CAD build for the part. Positions are in the model's coordinates, mm. A direction names the side the tool comes from. Coordinates: 2 decimals unless noted, no trailing zeros. Write each loop counter-clockwise with the first axis right and the second up, starting at its lowest first coordinate (ties: lowest second). Pieces come first, ordered by that corner, then holes. Notation, with made-up numbers: (81.25, 84.25) - (106.25, 84.25) arc R18 ccw to (106.25, 99.25) - close; hole circle Ø9 at (25, 47.25). An arc over 180 degrees is marked (long way). Answer in a Markdown table with one row per item. Add a question column.
Q1. 3-axis set-ups, long thin cutter, end or side, ignore diameter. For faces 1 (the flat face through (199, 0, 917)), 2 (the flat face through (373, 123, 1040)): which of +Z, -Z, +X, -X, +Y, -Y reach the whole face in a straight line?
Q2. Two-plate mould, pull along Z, no slides. Class faces 3 (the flat face through (203, 296, 1700)), 4 (the flat face through (101, 296, 200)), 5 (the flat face through (199, 600, 854)): +Z half, -Z half, draft (parallel to the pull), parting line (faces both ways), or undercut.
Q3. Band-saw the part on C-C (y = 512). State how many separate pieces and enclosed holes the cut face has, and give its area (3 significant figures).
Q4. Band-saw the part on A-A (x = 293). List the corners of the cut face in (y, z), and give its area (3 significant figures).
Q5. Band-saw the part on B-B (z = 1497.5). List the corners of the cut face in (x, y).
Q6. Pin check, flat tips, straight feed: pin 1 (1 mm diameter, centred on y = 376.5, z = 1068.5, fed in from -X); pin 2 (5 mm diameter, centred on x = 377, z = 545, fed in from +Y). Stop position of each tip, or through.
Q7. Drill centre lines: line 1 along Z through (x, y) = (384, 430.5); line 2 along X through (y, z) = (566, 227.5); line 3 along Z through (x, y) = (309.5, 558.5). Where is each one in solid material? Low to high. Write a range as from..to.
Autodesk Inventor part; units mm, degrees
ref_plane "YZ Plane" through (0, 0, 0) normal (1, 0, 0) x (0, 1, 0)
ref_plane "XZ Plane" through (0, 0, 0) normal (0, 1, 0) x (-1, 0, 0)
ref_plane "XY Plane" through (0, 0, 0) normal (0, 0, 1) x (1, 0, 0)
sketch "Sketch2" plane through (0, 0, 0) normal (0, 1, 0) x (-1, 0, 0)
  line L0 (-400, 180) -> (-400, 1700)
  line L1 (-400, 1700) -> (0, 1700)
  line L2 (0, 1700) -> (0, 180)
  line L3 (-400, 200) -> (-400, 600)
  line L4 (0, 600) -> (0, 200)
  line L5 (0, 600) -> (0, 700)
  line L6 (-400, 700) -> (-400, 600)
  line L7 (-400, 700) -> (-400, 1100)
  line L8 (0, 1100) -> (0, 700)
  line L9 (0, 1100) -> (0, 1200)
  line L10 (-400, 1200) -> (-400, 1100)
  line L11 (-400, 1200) -> (-400, 1600)
  line L12 (0, 1600) -> (0, 1200)
  line L13 (0, 200) -> (0, 180)
  line L14 (0, 180) -> (-400, 180)
  line L15 (-400, 180) -> (-400, 200)
  line L16 (0, 700) -> (0, 680)
  line L17 (-400, 680) -> (-400, 700)
  line L18 (0, 1200) -> (0, 1180)
  line L19 (-400, 1180) -> (-400, 1200)
  line L20 (-390, 200) -> (-210, 200)
  line L21 (-190, 200) -> (-10, 200)
  line L22 (-10, 200) -> (-190, 200)
  line L23 (-210, 200) -> (-390, 200)
  line L24 (-210, 680) -> (-210, 200)
  line L25 (-190, 680) -> (-190, 200)
  line L26 (-390, 700) -> (-210, 700)
  line L27 (-190, 700) -> (-10, 700)
  line L28 (-10, 700) -> (-190, 700)
  line L29 (-210, 700) -> (-390, 700)
  line L30 (-10, 700) -> (-190, 700)
  line L31 (-210, 700) -> (-390, 700)
  line L32 (-10, 680) -> (-190, 680)
  line L33 (-210, 680) -> (-390, 680)
  line L34 (-10, 680) -> (-10, 200)
  line L35 (-390, 200) -> (-390, 680)
  line L36 (-210, 1690) -> (-210, 1200)
  line L37 (-210, 1180) -> (-210, 700)
  line L38 (-190, 1690) -> (-190, 1200)
  line L39 (-190, 1180) -> (-190, 700)
  line L40 (-390, 1200) -> (-210, 1200)
  line L41 (-190, 1200) -> (-10, 1200)
  line L42 (-10, 1200) -> (-190, 1200)
  line L43 (-210, 1200) -> (-390, 1200)
  line L44 (-10, 1200) -> (-190, 1200)
  line L45 (-210, 1200) -> (-390, 1200)
  line L46 (-10, 1180) -> (-190, 1180)
  line L47 (-210, 1180) -> (-390, 1180)
  line L48 (-10, 1690) -> (-10, 1200)
  line L49 (-10, 1180) -> (-10, 700)
  line L50 (-390, 700) -> (-390, 1180)
  line L51 (-390, 1200) -> (-390, 1690)
  line L52 (-390, 1690) -> (-210, 1690)
  line L53 (-190, 1690) -> (-10, 1690)
  point P0 (0, 0)
  dimension "d0" = 400
  dimension "d6" = 400
  dimension "d7" = 100
  dimension "d8" = 400
  dimension "d9" = 400
  dimension "d10" = 100
  dimension "d11" = 400
  dimension "d12" = 400
  dimension "d14" = 400
  dimension "d15" = 20
  dimension "d16" = 20
  dimension "d17" = 20
  dimension "d25" = 10
extrude "Extrusion1" add sketch "Sketch2" along normal blind 600
sketch "Sketch3" plane through (400, 0, 180) normal (0, 0, -1) x (-1, 0, 0)
  line L0 (0, 0) -> (400, 0)
  line L1 (400, 0) -> (400, 600)
  line L2 (400, 600) -> (0, 600)
  line L3 (0, 600) -> (0, 0)
  line L4 (20, 300) -> (380, 300)
  line L5 (200, 0) -> (200, 600)
  line L6 (0, 0) -> (20, 0)
  line L7 (20, 0) -> (20, 600)
  line L8 (20, 600) -> (0, 600)
  line L9 (0, 600) -> (0, 0)
  line L10 (400, 600) -> (380, 600)
  line L11 (380, 600) -> (380, 0)
  line L12 (380, 0) -> (400, 0)
  line L13 (400, 0) -> (400, 600)
  dimension "d20" = 20
  dimension "d21" = 20
extrude "Extrusion2" add sketch "Sketch3" along normal blind 200 contours L3 L2 L7 L0 | L11 L2 L1 L0
sketch "Sketch4" plane through (10, 0, 680) normal (1, 0, 0) x (0, 0, -1)
  line L0 (0, 0) -> (480, 0)
  line L1 (130, 0) -> (130, 250)
  line L2 (130, 0) -> (380, 0) construction
  line L3 (130, 250) -> (140, 250)
  line L4 (140, 250) -> (140, 0)
  line L5 (130, 0) -> (140, 0)
  point P0 (680, 0)
  dimension "d26" = 250
  dimension "d27" = 90
  dimension "d28" = 10
extrude "Extrusion3" add sketch "Sketch4" along normal blind 35
sketch "Sketch5" plane through (10, 0, 1180) normal (1, 0, 0) x (0, 0, -1)
  line L0 (0, 0) -> (480, 0)
  line L1 (130, 0) -> (130, 250)
  line L2 (130, 0) -> (380, 0) construction
  line L3 (130, 250) -> (140, 250)
  line L4 (140, 250) -> (140, 0)
  line L5 (140, 0) -> (130, 0)
  line L6 (-510, 0) -> (-20, 0)
  line L7 (-370, 0) -> (-370, 250)
  line L8 (-370, 0) -> (-120, 0) construction
  line L9 (-370, 250) -> (-360, 250)
  line L10 (-360, 250) -> (-360, 0)
  line L11 (-360, 0) -> (-370, 0)
  point P0 (1180, 0)
  point P1 (-360, 0)
  dimension "d31" = 250
  dimension "d32" = 90
  dimension "d33" = 10
  dimension "d34" = 250
  dimension "d35" = 90
  dimension "d36" = 10
  dimension "d37" = 90
  dimension "d38" = 90
extrude "Extrusion4" add sketch "Sketch5" along normal blind 35
sketch "Sketch7" plane through (20, 0, 180) normal (1, 0, 0) x (0, 0, -1)
  line L0 (-1520, 0) -> (200, 0)
  line L1 (200, 0) -> (160, 0)
  line L2 (160, 0) -> (160, 600)
  line L3 (160, 600) -> (200, 600)
  line L4 (200, 600) -> (200, 0)
  point P0 (180, 0)
  point P1 (160, 0)
  dimension "d49" = 40
  dimension "d50" = 600
extrude "Extrusion6" add sketch "Sketch7" along normal blind 370
sketch "Sketch8" plane through (390, 0, 200) normal (-1, 0, 0) x (0, 0, 1)
  line L0 (1500, 0) -> (-220, 0)
  line L1 (350, 0) -> (340, 0)
  line L2 (340, 0) -> (340, 250)
  line L3 (340, 250) -> (350, 250)
  line L4 (350, 250) -> (350, 0)
  line L5 (850, 0) -> (840, 0)
  line L6 (840, 0) -> (840, 250)
  line L7 (840, 250) -> (850, 250)
  line L8 (850, 250) -> (850, 0)
  line L9 (1350, 0) -> (1340, 0)
  line L10 (1340, 0) -> (1340, 250)
  line L11 (1340, 250) -> (1350, 250)
  line L12 (1350, 250) -> (1350, 0)
  point P0 (-200, 0)
  dimension "d53" = 10
  dimension "d54" = 250
  dimension "d55" = 10
  dimension "d56" = 250
  dimension "d57" = 10
  dimension "d58" = 250
extrude "Extrusion7" add sketch "Sketch8" along normal blind 35
sketch "Sketch9" plane through (400, 0, -20) normal (0, 0, -1) x (-1, 0, 0)
  line L0 (400, 600) -> (0, 600)
  line L1 (400, 600) -> (0, 600)
  line L2 (0, 600) -> (0, 0)
  line L3 (0, 0) -> (400, 0)
  line L4 (400, 0) -> (400, 600)
  point P0 (400, 0)
extrude "Extrusion8" cut sketch "Sketch9" against normal blind 20
properties part number "MoldsStore"
Checked values:
| question | item | result |
|---|---|---|
| 1 | face 1 | +Z, -Z, +X, -X, -Y |
| 1 | face 2 | +Y, -Y |
| 2 | face 3 | +Z half |
| 2 | face 4 | undercut |
| 2 | face 5 | draft |
| 3 | separate pieces | 1 |
| 3 | enclosed holes | 7 |
| 3 | area | 100,000 mm² |
| 4 | outline | (0, 0) - (600, 0) - (600, 20) - (0, 20) - close; (0, 180) - (600, 180) - (600, 200) - (0, 200) - close; (0, 680) - (600, 680) - (600, 700) - (0, 700) - close; (0, 1180) - (600, 1180) - (600, 1200) - (0, 1200) - close; (0, 1690) - (600, 1690) - (600, 1700) - (0, 1700) - close |
| 4 | area | 54,000 mm² |
| 5 | outline | (0, 0) - (10, 0) - (10, 600) - (0, 600) - close; (190, 0) - (210, 0) - (210, 600) - (190, 600) - close; (390, 0) - (400, 0) - (400, 600) - (390, 600) - close |
| 6 | pin 1 | stops at x = 0 |
| 6 | pin 2 | stops at y = 250 |
| 7 | line 1 | z = 0..200, 680..700, 1180..1200, 1690..1700 |
| 7 | line 2 | x = 0..10, 190..210, 390..400 |
| 7 | line 3 | z = 0..20, 180..200, 680..700, 1180..1200, 1690..1700 |
